The model under review builds one solid part; all positions refer to its coordinate system, in mm. A direction names the side the tool comes from. Coordinates: 2 decimals unless noted, no trailing zeros. Loops run counter-clockwise (first coordinate to the right, second up) from the corner with the lowest first, then second, coordinate; pieces in that order, holes last. Notation, with made-up numbers: (81, -7) - (112, -7) arc R8 ccw to (112, 3) - close; hole circle Ø9 at (6.25, -14). An arc over 180 degrees is marked (long way). Use a Markdown table: item, result. Add a question column.
1) Add section B-B, the plane y = -4.25. Give the boundary of the cut face in (x, z), and give its area (3 significant figures).
2) To check wall thickness, follow L1, parallel to Y at x = 5, z = 0.75; L2, parallel to Y at x = -0.25, z = 4.5; L3, parallel to X at y = -0.5, z = 4.5. State the ranges of each line that lie inside material, in increasing order. Write a range as [from, to].
3) Add section D-D, the plane y = -0.5. Give the boundary of the cut face in (x, z), and give its area (3 significant figures).
4) The part is to be moulded in two halves that separate along X. For faces 1 (the flat face through (-0.775, -3, 4)), 2 (the flat face through (-3, -3, 3.153)), 3 (the cylindrical face through (-8.02, 0.74, 9.32)), 4 (the flat face through (-3, -6, 1)), say which applies: pulls with the +X half, pulls with the -X half, needs draft (parallel to the pull), parting line crosses it, or undercut.
5) For faces 5 (the flat face through (-1, 1, -4.397)), 6 (the flat face through (-3.325, -3, 3)), list the 3-axis set-ups (+Z, -Z, +X, -X, +Y, -Y) from which the entire face can be reached by the end or side of a thin tool; tool diameter is ignored.
6) Add section C-C, the plane z = 7.25. Give the boundary of the cut face in (x, y).
7) Add section A-A, the plane x = -5.25. Give the boundary of the cut face in (y, z), and give its area (3 significant figures).
8) Clearance check with flat-ended pins moving along their axes: pin 1 (3 mm diameter, centred on x = -1.5, y = -5, fed in from +Z); pin 2 (0.6 mm diameter, centred on y = -2.5, z = 3, fed in from +X); pin 3 (4 mm diameter, centred on x = 2, y = -2.5, fed in from -Z); pin 4 (5 mm diameter, centred on x = -2.5, y = -2, fed in from +Z). State where each tip first meets the part, or that it passes through.
```python
from build123d import *

# Parameters (mm, degrees)
BOSS_EXTRUDE1_DEPTH = 1.5
SKETCH2_R           = 2.75
BOSS_EXTRUDE2_DEPTH = 6
SKETCH3_W           = 1.1
SKETCH3_H           = 1.45
SKETCH3_W_2         = 1.45
SKETCH3_H_2         = 1.1
CUT_EXTRUDE1_DEPTH  = 6
CHAMFER1_SIZE       = 0.3
FILLET1_R           = 1
SKETCH4_R           = 1.25
BOSS_EXTRUDE3_DEPTH = 0.01
DOME1_FACE_RADIUS   = 1.25
DOME1_HEIGHT        = 1.25
FILLET3_R           = 0.2


with BuildPart() as part:
    # Sketch1 → Boss-Extrude1 (new body)
    with BuildSketch(Plane(origin=(0, 0, 0), x_dir=(1, 0, 0), z_dir=(0, 1, 0))):
        with BuildLine():
            Line((-7.324675649, 4.396717546), (4.675324351, 4.396717546))
            ThreePointArc((4.675324351, 4.396717546), (5.382431132, 4.103824327), (5.675324351, 3.396717546))
            Line((5.675324351, 3.396717546), (5.675324351, -8.603282454))
            ThreePointArc((5.675324351, -8.603282454), (5.382431132, -9.310389235), (4.675324351, -9.603282454))
            Line((4.675324351, -9.603282454), (-7.324675649, -9.603282454))
            ThreePointArc((-7.324675649, -9.603282454), (-8.03178243, -9.310389235), (-8.324675649, -8.603282454))
            Line((-8.324675649, -8.603282454), (-8.324675649, 3.396717546))
            ThreePointArc((-8.324675649, 3.396717546), (-8.03178243, 4.103824327), (-7.324675649, 4.396717546))
        make_face()
    extrude(amount=BOSS_EXTRUDE1_DEPTH)

    # Sketch2 → Boss-Extrude2 (add)
    with BuildSketch(Plane.XZ):
        with Locations(Location((-1.324675649, 2.603282454, 0), (0, 0, 270))):
            Circle(SKETCH2_R)
    extrude(amount=BOSS_EXTRUDE2_DEPTH)

    # Sketch3 → Cut-Extrude1 (cut)
    with BuildSketch(Plane.XZ.offset(6)):
        with Locations((-1.324675649, 3.878282454)):
            Rectangle(SKETCH3_W, SKETCH3_H)
        with Locations((-0.049675649, 2.603282454)):
            Rectangle(SKETCH3_W_2, SKETCH3_H_2)
        with Locations((-1.324675649, 2.603282454)):
            Rectangle(SKETCH3_W, SKETCH3_H_2)
        with Locations((-2.599675649, 2.603282454)):
            Rectangle(SKETCH3_W_2, SKETCH3_H_2)
        with Locations((-1.324675649, 1.328282454)):
            Rectangle(SKETCH3_W, SKETCH3_H)
    extrude(amount=-CUT_EXTRUDE1_DEPTH, mode=Mode.SUBTRACT)

    # Chamfer1
    chamfer1_edges = [part.edges().sort_by_distance(p)[0] for p in [
        (-0.774675649, -6, 3.878282454),
        (-0.049675649, -6, 3.153282454),
        (0.675324351, -6, 2.603282454),
        (-0.774675649, -6, 1.328282454),
        (-2.599675649, -6, 3.153282454),
        (-1.324675649, -6, 4.603282454),
        (-1.874675649, -6, 3.878282454),
        (-3.324675649, -6, 2.603282454),
        (-2.599675649, -6, 2.053282454),
        (-1.874675649, -6, 1.328282454),
        (-1.324675649, -6, 0.603282454),
        (-0.049675649, -6, 2.053282454),
    ]]
    chamfer(chamfer1_edges, length=CHAMFER1_SIZE)

    # Fillet1
    fillet1_edges = [part.edges().sort_by_distance(p)[0] for p in [
        (-1.324675649, 0, 5.353282454),
    ]]
    fillet(fillet1_edges, radius=FILLET1_R)

    # Sketch4 → Boss-Extrude3 (add)
    with BuildSketch(Plane(origin=(0, 1.5, 0), x_dir=(1, 0, 0), z_dir=(0, 1, 0))):
        with Locations(Location((-3.324675649, 1.396717546, 0), (0, 0, 90))):
            Circle(SKETCH4_R)
    extrude(amount=BOSS_EXTRUDE3_DEPTH)

    # Dome1: a dome of height H over a round flat face of radius A is a cap of a sphere of radius (A * A + H * H) / (2 * H)
    dome1_r = (DOME1_FACE_RADIUS * DOME1_FACE_RADIUS + DOME1_HEIGHT * DOME1_HEIGHT) / (2 * DOME1_HEIGHT)
    dome1_base = Plane((-3.324675649, 1.51, -1.396717546), z_dir=(0, 1, 0))
    with Locations(dome1_base.offset(DOME1_HEIGHT - dome1_r)):
        dome1_ball = Sphere(dome1_r, mode=Mode.PRIVATE)
    add(split(dome1_ball, bisect_by=dome1_base, keep=Keep.TOP, mode=Mode.PRIVATE))

    # Fillet3
    fillet3_edges = [part.edges().sort_by_distance(p)[0] for p in [
        (5.382431132, 1.5, 9.310389235),
        (-1.324675649, 0, 9.603282454),
        (-8.03178243, 0, 9.310389235),
        (5.675324351, 1.5, 2.603282454),
        (5.382431132, 1.5, -4.103824327),
        (-1.324675649, 1.5, -4.396717546),
        (-8.03178243, 1.5, -4.103824327),
        (-8.324675649, 1.5, 2.603282454),
        (-8.03178243, 1.5, 9.310389235),
        (-1.324675649, 1.5, 9.603282454),
        (-8.324675649, 0, 2.603282454),
        (-8.03178243, 0, -4.103824327),
        (-1.324675649, 0, -4.396717546),
        (5.382431132, 0, -4.103824327),
        (5.675324351, 0, 2.603282454),
        (5.382431132, 0, 9.310389235),
    ]]
    fillet(fillet3_edges, radius=FILLET3_R)


solid = part.part
```
From the geometry:
| question | item | result |
|---|---|---|
| 1 | outline | circle Ø5.5 at (-1.32, 2.6); hole (-3.32, 2.05) - (-1.87, 2.05) - (-1.87, 0.6) - (-0.77, 0.6) - (-0.77, 2.05) - (0.68, 2.05) - (0.68, 3.15) - (-0.77, 3.15) - (-0.77, 4.6) - (-1.87, 4.6) - (-1.87, 3.15) - (-3.32, 3.15) - close |
| 1 | area | 16.2 mm^2 |
| 2 | L1 | y = [0, 1.5] |
| 2 | L2 | y = [-6, 1.5] |
| 2 | L3 | x = [-3.5, -1.87], [-0.77, 0.85] |
| 3 | outline | circle Ø5.77 at (-1.32, 2.6); hole (-3.32, 2.05) - (-1.87, 2.05) - (-1.87, 0.6) - (-0.77, 0.6) - (-0.77, 2.05) - (0.68, 2.05) - (0.68, 3.15) - (-0.77, 3.15) - (-0.77, 4.6) - (-1.87, 4.6) - (-1.87, 3.15) - (-3.32, 3.15) - close |
| 3 | area | 18.5 mm^2 |
| 4 | face 1 | undercut |
| 4 | face 2 | undercut |
| 4 | face 3 | pulls with the -X half |
| 4 | face 4 | needs draft |
| 5 | face 5 | -Z, +X, -X, +Y, -Y |
| 5 | face 6 | -Y |
| 6 | outline | (-8.32, 0.2) arc R0.2 ccw to (-8.12, 0) - (5.48, 0) arc R0.2 ccw to (5.68, 0.2) - (5.68, 1.3) arc R0.2 ccw to (5.48, 1.5) - (-8.12, 1.5) arc R0.2 ccw to (-8.32, 1.3) - close |
| 7 | outline | (0, -4.2) arc R0.2 ccw to (0.2, -4.4) - (1.3, -4.4) arc R0.2 ccw to (1.5, -4.2) - (1.5, 9.4) arc R0.2 ccw to (1.3, 9.6) - (0.2, 9.6) arc R0.2 ccw to (0, 9.4) - close |
| 7 | area | 21.0 mm^2 |
| 8 | pin 1 | stops at z = 5.35 |
| 8 | pin 2 | stops at x = 1.42 |
| 8 | pin 3 | stops at z = 0.19 |
| 8 | pin 4 | stops at z = 9.6 |
